The model under review builds one solid part; all positions refer to its coordinate system, in mm. Round coordinates to 2 decimals unless told otherwise and drop trailing zeros. Return JSON: item names as keys, results as strings. Group by question number.
1. Clearance check with a flat-ended pin moving along its axis: P1, Ø4.5, axis at x = 38.06, z = 13.44, coming from the -Y side. State where the tip first meets the part, or that it passes through.
2. Take a section at A-A, the plane y = 0.7. Give the number of separate pieces and of enclosed holes in the cut face, then the cut area to 3 significant figures.
3. Mouldability with a two-part tool opening along X and no side actions: class faces 1 (the flat face through (15, 2, -43.259)), 2 (the cylindrical face through (13.148, 1.565, -7.62)) as pulls with the +X half, pulls with the -X half, needs draft (parallel to the pull), parting line crosses it, or undercut.
4. For line 1 along Z through (x, y) = (-2.5, 0.5); line 2 along Z through (x, y) = (62, 2.2); line 3 along Z through (x, y) = (-14.5, 1.1), list the stretches that pass through material, from the lowest coordinate up. Write a range as from..to.
from build123d import *

# Parameters (mm, degrees)
SKETCH1_W           = 156.35
SKETCH1_H           = 128
BOSS_EXTRUDE1_DEPTH = 3.175
SKETCH2_R           = 1.5
CUT_EXTRUDE1_DEPTH  = 10
SKETCH3_R           = 2.8575
CUT_EXTRUDE2_DEPTH  = 10


with BuildPart() as part:
    # Sketch1 → Boss-Extrude1 (new body)
    with BuildSketch(Plane(origin=(0, 0, 0), x_dir=(1, 0, 0), z_dir=(0, 1, 0))):
        with Locations((16.313207547, -20.741037736)):
            Rectangle(SKETCH1_W, SKETCH1_H)
    extrude(amount=BOSS_EXTRUDE1_DEPTH)

    # Sketch2 → Cut-Extrude1 (cut)
    with BuildSketch(Plane.XZ):
        with Locations((-21.186792453, 58.241037736)):
            Circle(SKETCH2_R)
        with Locations((53.813207547, 58.241037736)):
            Circle(SKETCH2_R)
        with Locations((53.813207547, -16.758962264)):
            Circle(SKETCH2_R)
        with Locations((-21.186792453, -16.758962264)):
            Circle(SKETCH2_R)
    extrude(amount=-CUT_EXTRUDE1_DEPTH, mode=Mode.SUBTRACT)

    # Sketch3 → Cut-Extrude2 (cut)
    with BuildSketch(Plane.XZ):
        with Locations((-6.178033112, 57.136048301)):
            Circle(SKETCH3_R)
        with Locations((2.821966888, 57.136048301)):
            Circle(SKETCH3_R)
        with Locations((11.821966888, 57.136048301)):
            Circle(SKETCH3_R)
        with Locations((20.821966888, 57.136048301)):
            Circle(SKETCH3_R)
        with Locations((29.821966888, 57.136048301)):
            Circle(SKETCH3_R)
        with Locations((38.821966888, 57.136048301)):
            Circle(SKETCH3_R)
        with Locations((-10.513543723, 50.195532798)):
            Circle(SKETCH3_R)
        with Locations((-1.513543723, 50.195532798)):
            Circle(SKETCH3_R)
        with Locations((7.486456277, 50.195532798)):
            Circle(SKETCH3_R)
        with Locations((16.486456277, 50.195532798)):
            Circle(SKETCH3_R)
        with Locations((25.486456277, 50.195532798)):
            Circle(SKETCH3_R)
        with Locations((34.486456277, 50.195532798)):
            Circle(SKETCH3_R)
        with Locations((43.486456277, 50.195532798)):
            Circle(SKETCH3_R)
        with Locations((-15.52660687, 42.439711518)):
            Circle(SKETCH3_R)
        with Locations((-6.52660687, 42.439711518)):
            Circle(SKETCH3_R)
        with Locations((2.47339313, 42.439711518)):
            Circle(SKETCH3_R)
        with Locations((11.47339313, 42.439711518)):
            Circle(SKETCH3_R)
        with Locations((20.47339313, 42.439711518)):
            Circle(SKETCH3_R)
        with Locations((29.47339313, 42.439711518)):
            Circle(SKETCH3_R)
        with Locations((38.47339313, 42.439711518)):
            Circle(SKETCH3_R)
        with Locations((47.47339313, 42.439711518)):
            Circle(SKETCH3_R)
        with Locations((-19.862117481, 35.499196015)):
            Circle(SKETCH3_R)
        with Locations((-10.862117481, 35.499196015)):
            Circle(SKETCH3_R)
        with Locations((-1.862117481, 35.499196015)):
            Circle(SKETCH3_R)
        with Locations((34.137882519, 35.499196015)):
            Circle(SKETCH3_R)
        with Locations((43.137882519, 35.499196015)):
            Circle(SKETCH3_R)
        with Locations((52.137882519, 35.499196015)):
            Circle(SKETCH3_R)
        with Locations((-24.594118133, 28.137585821)):
            Circle(SKETCH3_R)
        with Locations((-15.594118133, 28.137585821)):
            Circle(SKETCH3_R)
        with Locations((-6.594118133, 28.137585821)):
            Circle(SKETCH3_R)
        with Locations((38.405881867, 28.137585821)):
            Circle(SKETCH3_R)
        with Locations((47.405881867, 28.137585821)):
            Circle(SKETCH3_R)
        with Locations((56.405881867, 28.137585821)):
            Circle(SKETCH3_R)
        with Locations((-28.929628744, 21.197070319)):
            Circle(SKETCH3_R)
        with Locations((-19.929628744, 21.197070319)):
            Circle(SKETCH3_R)
        with Locations((-10.929628744, 21.197070319)):
            Circle(SKETCH3_R)
        with Locations((43.070371256, 21.197070319)):
            Circle(SKETCH3_R)
        with Locations((52.070371256, 21.197070319)):
            Circle(SKETCH3_R)
        with Locations((-24.942691891, 13.441249039)):
            Circle(SKETCH3_R)
        with Locations((-15.942691891, 13.441249039)):
            Circle(SKETCH3_R)
        with Locations((-6.942691891, 13.441249039)):
            Circle(SKETCH3_R)
        with Locations((38.057308109, 13.441249039)):
            Circle(SKETCH3_R)
        with Locations((47.057308109, 13.441249039)):
            Circle(SKETCH3_R)
        with Locations((56.057308109, 13.441249039)):
            Circle(SKETCH3_R)
        with Locations((-20.278202502, 6.500733536)):
            Circle(SKETCH3_R)
        with Locations((-11.278202502, 6.500733536)):
            Circle(SKETCH3_R)
        with Locations((-2.278202502, 6.500733536)):
            Circle(SKETCH3_R)
        with Locations((33.721797498, 6.500733536)):
            Circle(SKETCH3_R)
        with Locations((42.721797498, 6.500733536)):
            Circle(SKETCH3_R)
        with Locations((51.721797498, 6.500733536)):
            Circle(SKETCH3_R)
        with Locations((-15.662214589, -0.805516952)):
            Circle(SKETCH3_R)
        with Locations((-6.662214589, -0.805516952)):
            Circle(SKETCH3_R)
        with Locations((2.337785411, -0.805516952)):
            Circle(SKETCH3_R)
        with Locations((11.337785411, -0.805516952)):
            Circle(SKETCH3_R)
        with Locations((20.337785411, -0.805516952)):
            Circle(SKETCH3_R)
        with Locations((29.337785411, -0.805516952)):
            Circle(SKETCH3_R)
        with Locations((38.337785411, -0.805516952)):
            Circle(SKETCH3_R)
        with Locations((47.337785411, -0.805516952)):
            Circle(SKETCH3_R)
        with Locations((-10.9977252, -7.746032454)):
            Circle(SKETCH3_R)
        with Locations((-1.9977252, -7.746032454)):
            Circle(SKETCH3_R)
        with Locations((7.0022748, -7.746032454)):
            Circle(SKETCH3_R)
        with Locations((16.0022748, -7.746032454)):
            Circle(SKETCH3_R)
        with Locations((25.0022748, -7.746032454)):
            Circle(SKETCH3_R)
        with Locations((34.0022748, -7.746032454)):
            Circle(SKETCH3_R)
        with Locations((43.0022748, -7.746032454)):
            Circle(SKETCH3_R)
        with Locations((-6.137528578, -15.018990423)):
            Circle(SKETCH3_R)
        with Locations((2.862471422, -15.018990423)):
            Circle(SKETCH3_R)
        with Locations((11.862471422, -15.018990423)):
            Circle(SKETCH3_R)
        with Locations((20.862471422, -15.018990423)):
            Circle(SKETCH3_R)
        with Locations((29.862471422, -15.018990423)):
            Circle(SKETCH3_R)
        with Locations((38.862471422, -15.018990423)):
            Circle(SKETCH3_R)
        with Locations((61.811516702, 21.197070319)):
            Circle(SKETCH3_R)
    extrude(amount=-CUT_EXTRUDE2_DEPTH, mode=Mode.SUBTRACT)


solid = part.part
Output:
{
 "1": {"P1": "passes through"},
 "2": {"separate pieces": "1", "enclosed holes": "76", "area": "18,100 mm^2"},
 "3": {"face 1": "needs draft", "face 2": "undercut"},
 "4": {"line 1": "z = -43.26..-10.56, -4.93..3.65, 9.35..32.71, 38.28..47.51, 52.88..84.74", "line 2": "z = -43.26..18.35, 24.05..84.74", "line 3": "z = -43.26..-3.42, 1.8..10.97, 15.91..25.5, 30.78..39.77, 45.11..84.74"}
}
